Could you check a few things on this model? Use its own coordinates, in mm. A direction names the side the tool comes from. Coordinates: 2 decimals unless noted, no trailing zeros. Order: outer loops, then holes, each group sorted by start corner. A loop starts at its lowest first (then second) coordinate and runs counter-clockwise, first axis right, second up. Notation, with made-up numbers: M 16,-27.75 L 47,-27.75 A32 cw 47,6.25 Z; hole C 83,64.5 d7. An arc over 180 degrees is marked long. Put each result on its own line as item: value. Start each with the question number.
```python
from build123d import *

# Parameters (mm, degrees)
BOSS_EXTRU_1_DEPTH = 1
ESQUISSE2_W        = 28.5
ESQUISSE2_H        = 54.569597512
ESQUISSE2_W_2      = 26.5
ESQUISSE2_H_2      = 52.569597512
BOSS_EXTRU_2_DEPTH = 4


with BuildPart() as part:
    # Esquisse1 → Boss.-Extru.1 (new body)
    with BuildSketch(Plane.XY):
        with BuildLine():
            Line((0, 27.569597512), (0, 0))
            Line((0, 0), (4, 0))
            Line((4, 0), (4, 23.569597512))
            ThreePointArc((4, 23.569597512), (5.464466094, 27.105131417), (9, 28.569597512))
            Line((9, 28.569597512), (47.9850382, 28.569597512))
            Line((47.9850382, 28.569597512), (47.9850382, 17))
            Line((47.9850382, 17), (51.319537583, 17))
            Line((51.319537583, 17), (51.319537583, 0))
            Line((51.319537583, 0), (52.319537583, 0))
            Line((52.319537583, 0), (53.567879902, 12.496984059))
            ThreePointArc((53.567879902, 12.496984059), (55.187893525, 15.707082431), (58.543119277, 17))
            Line((58.543119277, 17), (65.935302341, 17))
            ThreePointArc((65.935302341, 17), (69.290528094, 15.707082431), (70.910541717, 12.496984059))
            Line((70.910541717, 12.496984059), (72.158884036, 0))
            Line((72.158884036, 0), (73.158884036, 0))
            Line((73.158884036, 0), (73.158884036, 17))
            Line((73.158884036, 17), (76.4850382, 17))
            Line((76.4850382, 17), (76.4850382, 28.569597512))
            Line((76.4850382, 28.569597512), (115.4700764, 28.569597512))
            ThreePointArc((115.4700764, 28.569597512), (119.005610306, 27.105131417), (120.4700764, 23.569597512))
            Line((120.4700764, 23.569597512), (120.4700764, 0))
            Line((120.4700764, 0), (125.415873255, 0))
            Line((125.415873255, 0), (125.415873255, 27.569597512))
            ThreePointArc((125.415873255, 27.569597512), (123.951407161, 31.105131417), (120.415873255, 32.569597512))
            Line((120.415873255, 32.569597512), (76.4850382, 32.569597512))
            Line((76.4850382, 32.569597512), (76.4850382, 71.569597512))
            Line((76.4850382, 71.569597512), (47.9850382, 71.569597512))
            Line((47.9850382, 71.569597512), (47.9850382, 32.569597512))
            Line((47.9850382, 32.569597512), (5, 32.569597512))
            ThreePointArc((5, 32.569597512), (1.464466094, 31.105131417), (0, 27.569597512))
        make_face()
    extrude(amount=BOSS_EXTRU_1_DEPTH)

    # Esquisse2 → Boss.-Extru.2 (add)
    with BuildSketch(Plane.XY.offset(1)):
        with Locations((62.2350382, 44.284798756)):
            Rectangle(ESQUISSE2_W, ESQUISSE2_H)
        with Locations((62.2350382, 44.284798756)):
            Rectangle(ESQUISSE2_W_2, ESQUISSE2_H_2, mode=Mode.SUBTRACT)
    extrude(amount=BOSS_EXTRU_2_DEPTH)


solid = part.part
```
Item 1: If we mould it in two halves opening along X, with no side actions, what happens to faces 1 (the cylindrical face through (69.3, 15.7, 0.5)), 2 (the cylindrical face through (123.99, 31.066, 0.493)), 3 (the cylindrical face through (1.5, 31.14, 0.49)), 4 (the flat face through (76, 52, 5))? For each: released by +X, released by -X, zero draft, split by the parting line, or undercut.
Item 2: I need wall thicknesses on probe 1 along X at (y, z) = (46, 1.7); probe 2 along Y at (x, z) = (74, 3.6); probe 3 along X at (y, z) = (45, 0.6). Which ranges of each line are inside material? Lowest first, please.
Item 3: If we section it at A-A on z = 2.7: Write out the boundary of the cut face in (x, y).
Item 4: If we section it at C-C on y = 44.5: Write out the boundary of the cut face in (x, z).
Item 5: If we section it at B-B on y = 4.5: Write out the boundary of the cut face in (x, z).
Item 6: If we section it at D-D on x = 43: Write out the boundary of the cut face in (y, z), then the cut area to 3 significant figures.
Item 7: For pin 1 Ø0.8 at (x, z) = (26, 0.5) entering from +Y; pin 2 Ø12 at (x, y) = (63, 24.5) entering from +Z; pin 3 Ø1.1 at (x, z) = (91, 0.5) entering from -Y, each with a flat end and sliding along its axis, tell me the tip position at first contact or that it passes through.
Item 8: For faces 5 (the flat face through (114, 30, 1)), 6 (the flat face through (53, 10, 1)), 7 (the flat face through (15, 30, 1)), which set-ups out of +Z, -Z, +X, -X, +Y, -Y let a thin tool reach every point of the face, with its end or its side?
Geometry check:
1. face 1: undercut
1. face 2: released by +X
1. face 3: released by -X
1. face 4: zero draft
2. probe 1: x = 47.99 to 48.99, 75.49 to 76.49
2. probe 2: y = 17 to 18, 70.57 to 71.57
2. probe 3: x = 47.99 to 76.49
3. outline: M 47.99,17 L 76.49,17 L 76.49,71.57 L 47.99,71.57 Z; hole M 48.99,18 L 75.49,18 L 75.49,70.57 L 48.99,70.57 Z
4. outline: M 47.99,0 L 76.49,0 L 76.49,5 L 75.49,5 L 75.49,1 L 48.99,1 L 48.99,5 L 47.99,5 Z
5. outline: M 0,0 L 4,0 L 4,1 L 0,1 Z; M 51.32,0 L 52.77,0 L 52.77,1 L 51.32,1 Z; M 71.71,0 L 73.16,0 L 73.16,1 L 71.71,1 Z; M 120.47,0 L 125.42,0 L 125.42,1 L 120.47,1 Z
6. outline: M 28.57,0 L 32.57,0 L 32.57,1 L 28.57,1 Z
6. area: 4.00 mm²
7. pin 1: stops at y = 32.57
7. pin 2: stops at z = 1
7. pin 3: stops at y = 28.57
8. face 5: +Z, +X, +Y, -Y
8. face 6: +Z, +X, -X, -Y
8. face 7: +Z, -X, +Y, -Y
